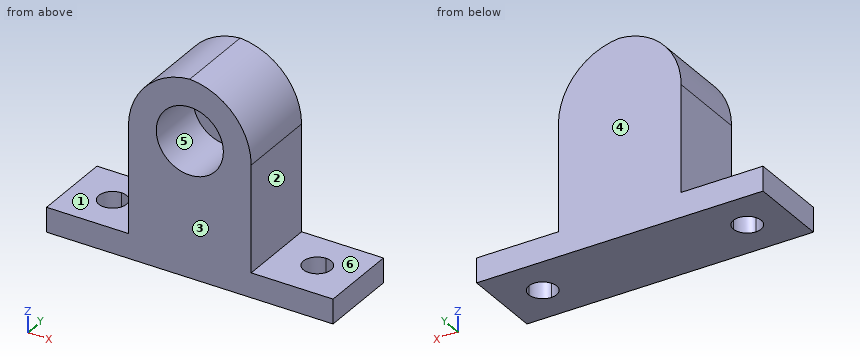
from build123d import *

# Parameters (mm, degrees)
BOSS_EXTRUDE1_DEPTH = 3
SKETCH2_W           = 15
SKETCH2_H           = 21.14750363
BOSS_EXTRUDE2_DEPTH = 9.822712027
FILLET1_R           = 8
CUT_EXTRUDE1_START  = -7.2
SKETCH3_R           = 4.1
CUT_EXTRUDE1_DEPTH  = 7.2


with BuildPart() as part:
    # Sketch1 → Boss-Extrude1 (new body)
    with BuildSketch(Plane.XY):
        with BuildLine():
            Line((-241.35, 304.622712027), (-266.35, 304.622712027))
            Line((-266.35, 304.622712027), (-266.35, 301.411356013))
            ThreePointArc((-266.35, 301.411356013), (-265.147918472, 300.913437541), (-264.65, 299.711356013))
            ThreePointArc((-264.65, 299.711356013), (-265.147918472, 298.509274485), (-266.35, 298.011356013))
            Line((-266.35, 298.011356013), (-266.35, 294.8))
            Line((-266.35, 294.8), (-241.35, 294.8))
            Line((-241.35, 294.8), (-241.35, 298.011356013))
            ThreePointArc((-241.35, 298.011356013), (-243.05, 299.711356013), (-241.35, 301.411356013))
            Line((-241.35, 301.411356013), (-241.35, 304.622712027))
        make_face()
        with BuildLine():
            Line((-266.35, 304.622712027), (-271.35, 304.622712027))
            Line((-271.35, 304.622712027), (-271.35, 294.8))
            Line((-271.35, 294.8), (-269.799999998, 294.8))
            Line((-269.799999998, 294.8), (-266.35, 294.8))
            Line((-266.35, 294.8), (-266.35, 298.011356013))
            ThreePointArc((-266.35, 298.011356013), (-268.05, 299.711356013), (-266.35, 301.411356013))
            Line((-266.35, 301.411356013), (-266.35, 304.622712027))
        make_face()
        with BuildLine():
            Line((-236.35, 304.622712027), (-241.35, 304.622712027))
            Line((-241.35, 304.622712027), (-241.35, 301.411356013))
            ThreePointArc((-241.35, 301.411356013), (-240.147918472, 300.913437541), (-239.65, 299.711356013))
            ThreePointArc((-239.65, 299.711356013), (-240.147918472, 298.509274485), (-241.35, 298.011356013))
            Line((-241.35, 298.011356013), (-241.35, 294.8))
            Line((-241.35, 294.8), (-236.35, 294.8))
            Line((-236.35, 294.8), (-236.35, 304.622712027))
        make_face()
    extrude(amount=BOSS_EXTRUDE1_DEPTH)

    # Sketch2 → Boss-Extrude2 (add)
    with BuildSketch(Plane(origin=(0, 304.622712027, 0), x_dir=(1, 0, 0), z_dir=(0, 1, 0))):
        with Locations((-253.85, -13.407165318)):
            Rectangle(SKETCH2_W, SKETCH2_H)
    extrude(amount=-BOSS_EXTRUDE2_DEPTH)

    # Fillet1
    # the kernel refuses this fillet: 8 mm, written as the material it takes off along each edge
    with BuildSketch(Plane(origin=(-246.35, 324.622712027, 23.980917133), x_dir=(0, 0, -1), z_dir=(0, -1, 0))) as fillet1_piece_1:
        with BuildLine():
            CenterArc((FILLET1_R, -FILLET1_R), FILLET1_R, 90, 90)
            Line((0, -FILLET1_R), (0, 0))
            Line((0, 0), (FILLET1_R, 0))
        make_face()
    extrude(amount=49.822712027, mode=Mode.SUBTRACT)
    with BuildSketch(Plane(origin=(-261.35, 324.622712027, 23.980917133), x_dir=(0, 0, -1), z_dir=(0, -1, 0))) as fillet1_piece_2:
        with BuildLine():
            CenterArc((FILLET1_R, FILLET1_R), FILLET1_R, 180, 90)
            Line((0, FILLET1_R), (0, 0))
            Line((0, 0), (FILLET1_R, 0))
        make_face()
    extrude(amount=49.822712027, mode=Mode.SUBTRACT)

    # Sketch3 → Cut-Extrude1 (cut)
    with BuildSketch(Plane.XZ.offset(-294.8).offset(CUT_EXTRUDE1_START)):
        with Locations((-253.85, 16.5)):
            Circle(SKETCH3_R)
    extrude(amount=CUT_EXTRUDE1_DEPTH, mode=Mode.SUBTRACT)


solid = part.part
Design review of the part built by this model. Coordinates are the model's own, in mm. Face numbers are marked on the shaded views. A direction names the side the tool comes from. Coordinates: 2 decimals unless noted, no trailing zeros. Loops run counter-clockwise (first coordinate to the right, second up) from the corner with the lowest first, then second, coordinate; pieces in that order, holes last. Notation, with made-up numbers: M 56,30.25 L 94,30.25 A24 cw 94,54.25 Z; hole C -36.5,1.25 d10. An arc over 180 degrees is marked long. Answer as CSV lines item,"result".
Item 1: Add section D-D on y = 304. State the section outline as (x, z) points, plus the area to 3 significant figures.
Answer list:
outline,"M -271.35,0 L -236.35,0 L -236.35,3 L -246.35,3 L -246.35,15.98 A8 ccw -253.85,23.97 A8 ccw -261.35,15.98 L -261.35,3 L -271.35,3 Z"
area,"392 mm²"
Item 2: The part is to be moulded in two halves that separate along Z. For the marked faces 4, 5 and 6, say which applies: pulls with the +Z half, pulls with the -Z half, needs draft (parallel to the pull), parting line crosses it, or undercut.
Answer list:
face 4,"needs draft"
face 5,"undercut"
face 6,"pulls with the +Z half"
Item 3: Add section B-B on y = 296.75. State the section outline as (x, z) points, plus the area to 3 significant figures.
Answer list:
outline,"M -271.35,0 L -236.35,0 L -236.35,3 L -246.35,3 L -246.35,15.98 A8 ccw -253.85,23.97 A8 ccw -261.35,15.98 L -261.35,3 L -271.35,3 Z; hole C -253.85,16.5 d8.2"
area,"339 mm²"
Item 4: Add section A-A on y = 300.5. State the section outline as (x, z) points, plus the area to 3 significant figures.
Answer list:
outline,"M -271.35,0 L -267.86,0 L -267.86,3 L -271.35,3 Z; M -264.84,0 L -242.86,0 L -242.86,3 L -246.35,3 L -246.35,15.98 A8 ccw -253.85,23.97 A8 ccw -261.35,15.98 L -261.35,3 L -264.84,3 Z; M -239.84,0 L -236.35,0 L -236.35,3 L -239.84,3 Z; hole C -253.85,16.5 d8.2"
area,"321 mm²"
Item 5: For P1, Ø3, axis at x = -244, y = 299, coming from the +Z side; P2, Ø1.5, axis at y = 299, z = 8.5, coming from the -X side; P3, Ø5, axis at x = -257.5, y = 302, coming from the +Z side, all flat-tipped, find the tip position at first contact; note any pin that passes through.
Answer list:
P1,"z = 3"
P2,"x = -261.35"
P3,"z = 23.81"
Item 6: Machinability: for the marked faces 1, 2 and 3, which of the approach directions +Z, -Z, +X, -X, +Y, -Y give a long, thin tool a straight path to every point of the face, cutting with its end or side? Answer none if there is none.
Answer list:
face 1,"+Z, -X, +Y, -Y"
face 2,"+Z, +X, +Y, -Y"
face 3,"+Z, -Z, +X, -X, -Y"
Item 7: Add section C-C on z = 2. State the section outline as (x, y) points, plus the area to 3 significant figures.
Answer list:
outline,"M -271.35,294.8 L -236.35,294.8 L -236.35,304.62 L -271.35,304.62 Z; hole C -266.35,299.71 d3.4; hole C -241.35,299.71 d3.4"
area,"326 mm²"
Item 8: For probe 1 along Z at (x, y) = (-253.85, 299.5); probe 2 along X at (y, z) = (299.5, 1.5); probe 3 along X at (y, z) = (296, 11), list the stretches that pass through material, from the lowest coordinate up.
Answer list:
probe 1,"0 to 12.4, 20.6 to 23.97"
probe 2,"-271.35 to -268.04, -264.66 to -243.04, -239.66 to -236.35"
probe 3,"-261.35 to -246.35"
